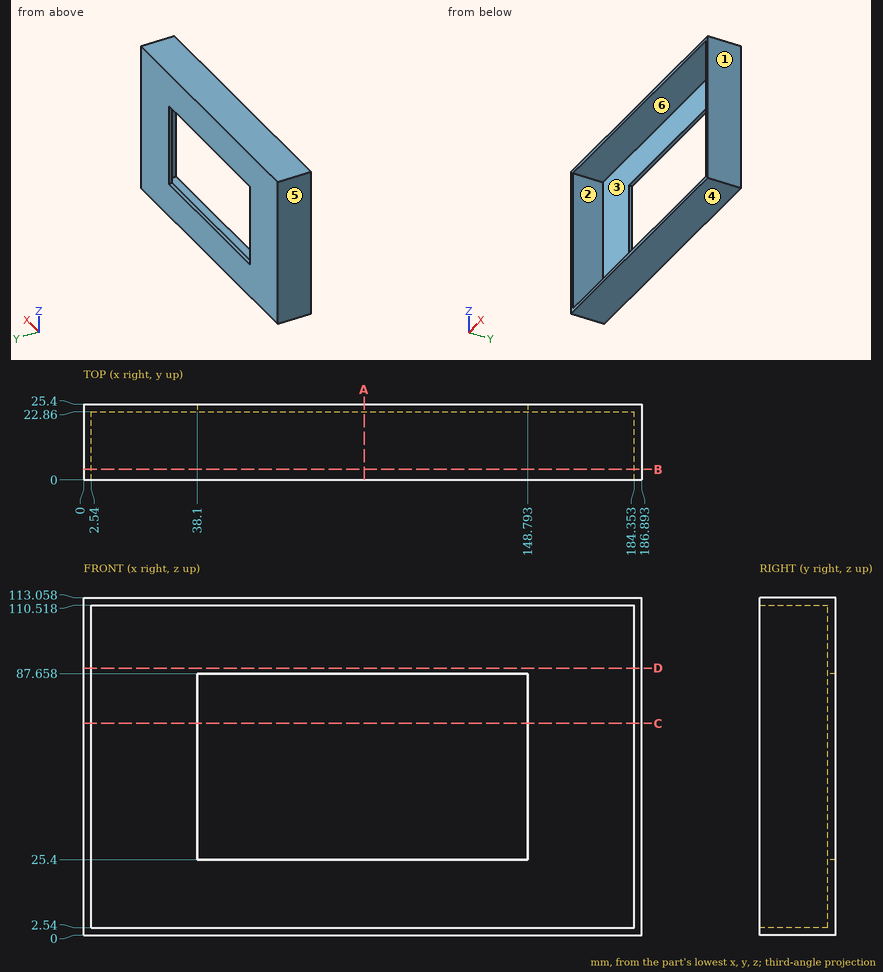
Part print with two shaded views. Sizes in mm from the minimum x, y, z corner. A direction names the side the tool comes from. Give positions to 0.01 mm unless a question says otherwise; leave off trailing zeros. Order: outer loops, then holes, each group sorted by start corner. A loop starts at its lowest first (then second) coordinate and runs counter-clockwise, first axis right, second up. Notation, with made-up numbers: M 47.5,66 L 89.5,66 A9 cw 89.5,81 Z; hole C -11.5,75.25 d8. An arc over 180 degrees is marked long. Put each result on its own line as item: value.
Item 1: Which spindle directions (+Z, -Z, +X, -X, +Y, -Y) get a long thin tool onto all of the face, cutting with end or side? Do the marked faces 5 and 6. Say none if no direction does.
Results are:
face 5: +Z, -Z, -X, +Y, -Y
face 6: -Y
Item 2: Drop a flat-ended pin along its axis: pin 1 Ø3 at (y, z) = (5.5, 43) entering from -X. Give the stop position or say it passes through.
Results are:
pin 1: x = 0
Item 3: Cut at B-B on y = 3.5. Write the cut outline in (x, z), then the cut area to 3 significant figures.
Results are:
outline: M 0,0 L 186.89,0 L 186.89,113.06 L 0,113.06 Z; hole M 2.54,2.54 L 184.35,2.54 L 184.35,110.52 L 2.54,110.52 Z
area: 1,500 mm2
Item 4: Pull direction Z, two halves, no side cores. Call the marked faces 1, 2, 3 and 4: +Z half, -Z half, draft (parallel to the pull), parting line (faces both ways), or undercut.
Results are:
face 1: draft
face 2: undercut
face 3: undercut
face 4: -Z half
Item 5: Cut at C-C on z = 71. Write the cut outline in (x, y), then the cut area to 3 significant figures.
Results are:
outline: M 0,0 L 2.54,0 L 2.54,22.86 L 38.1,22.86 L 38.1,25.4 L 0,25.4 Z; M 148.79,22.86 L 184.35,22.86 L 184.35,0 L 186.89,0 L 186.89,25.4 L 148.79,25.4 Z
area: 310 mm2
Item 6: Wall check: probe 1 along X at (y, z) = (2.5, 91); probe 2 along X at (y, z) = (24, 45.5); probe 3 along Z at (x, y) = (141, 1.25). Give the ranges that are in metal, low to high.
Results are:
probe 1: 0 to 2.54, 184.35 to 186.89
probe 2: 0 to 38.1, 148.79 to 186.89
probe 3: 0 to 2.54, 110.52 to 113.06
Item 7: Cut at A-A on x = 94. Write the cut outline in (y, z), then the cut area to 3 significant figures.
Results are:
outline: M 0,0 L 25.4,0 L 25.4,25.4 L 22.86,25.4 L 22.86,2.54 L 0,2.54 Z; M 0,110.52 L 22.86,110.52 L 22.86,87.66 L 25.4,87.66 L 25.4,113.06 L 0,113.06 Z
area: 245 mm2
Item 8: Cut at D-D on z = 89.5. Write the cut outline in (x, y).
Results are:
outline: M 0,0 L 2.54,0 L 2.54,22.86 L 184.35,22.86 L 184.35,0 L 186.89,0 L 186.89,25.4 L 0,25.4 Z
